Geometry: final body of the model. Coordinates: model frame, mm. A direction names the side the tool comes from. Round coordinates to 2 decimals unless told otherwise and drop trailing zeros. Order: outer loops, then holes, each group sorted by start corner. A loop starts at its lowest first (then second) coordinate and runs counter-clockwise, first axis right, second up. Notation, with made-up numbers: (74.5, 20.5) - (122.5, 20.5) arc R9 cw to (122.5, 24.5) - close; hole circle Ø6 at (-26, 27). An arc over 180 degrees is marked (long way). Put each result on its own line as item: value. Start each with the question number.
(1) Section C-C (y = 34). Output: boundary loops of the cut face in (x, z).
(2) Access query for faces 1 (the face through (0, 0, 4)), 2 (the face through (0.13, -1.93, 2.52)), 3 (the face through (0, 0, -4)). Directions: +Z, -Z, +X, -X, +Y, -Y. A direction counts if a zero-diameter tool reaches every point of the face in a straight line with its end or side. Return the directions, or none.
(3) Section D-D (x = -6.5). Output: boundary loops of the cut face in (y, z) (3 decimals), and give its area (3 significant figures).
(4) Pin query (flat end, axial travel): P1, Ø1.5, axis at x = -13, z = -0.5, coming from the +Y side; P2, Ø0.6, axis at x = 1, z = 4.5, coming from the -Y side; P3, Ø3.5, axis at x = 13, z = 0.5, coming from the +Y side. Return the tip coordinate at first contact, or that it passes through.
(5) Material intervals for L1, parallel to Y at x = -11.75, z = -2.25; L2, parallel to X at y = 14.5, z = -3.75; L3, parallel to Y at x = -7.75, z = 2.5, sorted ascending. Write a range as [from, to].
from build123d import *

# Parameters (mm, degrees)
SKETCH3_R           = 3.175
BOSS_EXTRUDE1_DEPTH = 12.7
FILLET1_R           = 3.175
SKETCH4_W           = 5.08
SKETCH4_H           = 1.524
BOSS_EXTRUDE2_DEPTH = 14.2875
SKETCH5_R           = 1.5875
BOSS_EXTRUDE3_DEPTH = 6.35
DRAFT1_ANGLE        = 5


with BuildPart() as part:
    # Sketch1 → Revolve1 (revolve)
    with BuildSketch(Plane.XY, mode=Mode.PRIVATE) as revolve1_sk:
        Polygon((0, 50.8), (0, 0), (5.075315188, 0), (2.413, 50.8), align=None)
    revolve(revolve1_sk.sketch.rotate(Axis((0, 50.8, 0), (0, -1, 0)), 180), axis=Axis((0, 50.8, 0), (0, -1, 0)))

    # Sketch3 → Boss-Extrude1 (add, symmetric)
    with BuildSketch(Plane(origin=(0, 0, 0), x_dir=(0, 0, -1), z_dir=(1, 0, 0))):
        Circle(SKETCH3_R)
    extrude(amount=BOSS_EXTRUDE1_DEPTH, both=True)

    # Fillet1
    fillet1_edges = [part.edges().sort_by_distance(p)[0] for p in [
        (-12.7, 0, 3.175),
        (12.7, 0, 3.175),
    ]]
    fillet(fillet1_edges, radius=FILLET1_R)

    # Sketch4 → Boss-Extrude2 (add, symmetric)
    with BuildSketch(Plane(origin=(0, 0, 0), x_dir=(0, 0, -1), z_dir=(1, 0, 0))):
        Rectangle(SKETCH4_W, SKETCH4_H)
    extrude(amount=BOSS_EXTRUDE2_DEPTH, both=True)

    # Sketch5 → Boss-Extrude3 (add)
    with BuildSketch(Plane(origin=(0, 0, 0), x_dir=(1, 0, 0), z_dir=(0, 1, 0))):
        with Locations(Location((0, 0, 0), (0, 0, 270))):
            Circle(SKETCH5_R)
    extrude(amount=-BOSS_EXTRUDE3_DEPTH)

    # Draft1
    draft1_faces = [part.faces().sort_by_distance(p)[0] for p in [
        (0, -4.549815329, -1.5875),
    ]]
    draft(draft1_faces, Plane(origin=(0, -6.35, 0), x_dir=(0, 0, -1), z_dir=(0, -1, 0)), DRAFT1_ANGLE)


solid = part.part
Checks:
1. outline: circle Ø6.59 at (0, 0)
2. face 1: +Z, +X, -X, -Y
2. face 2: none
2. face 3: -Z, +X, -X, -Y
3. outline: circle Ø6.35 at (0, 0)
3. area: 31.7 mm²
4. P1: stops at y = 1.57
4. P2: stops at y = 0
4. P3: stops at y = 2.64
5. L1: y = [-0.76, 0.76]
5. L2: x = [-2.14, 2.14]
5. L3: y = [-1.96, 1.96]
